Check sheet for the modelled part. Datum: model origin and axes. Units: mm. Coordinates: 2 decimals unless noted, no trailing zeros. Loops run counter-clockwise (first coordinate to the right, second up) from the corner with the lowest first, then second, coordinate; pieces in that order, holes last. Notation, with made-up numbers: (17, 29) - (60, 29) arc R23 ccw to (60, 49) - close; hole circle Ø6 at (17.5, -22). An arc over 180 degrees is marked (long way). Write each question's results on one line, items separated by ' | '. Start each with the question number.
1. Cross-section at A-A (x = 11.5). Record the cut outline in (y, z), and give its area (3 significant figures).
2. Thickness scan on line 1 (Z direction, x = 4, y = 6.5); line 2 (Z direction, x = 10, y = 7); line 3 (X direction, y = 3.75, z = -44.5). Record the ranges inside material, lowest first. Write a range as [from, to].
3. Cross-section at C-C (y = 3.75). Record the cut outline in (x, z).
4. Cross-section at B-B (z = -42). Record the cut outline in (x, y).
5. Cross-section at D-D (x = 3.5). Record the cut outline in (y, z), and give its area (3 significant figures).
```python
from build123d import *

# Parameters (mm, degrees)
SKETCH1_R           = 7
BOSS_EXTRUDE1_DEPTH = 8


with BuildPart() as part:
    # Sketch1 → Boss-Extrude1 (new body)
    with BuildSketch(Plane(origin=(0, 0, 0), x_dir=(1, 0, 0), z_dir=(0, 1, 0))):
        with BuildLine():
            Line((45.232378219, 82.321586231), (45.232378219, -94.678413769))
            Line((45.232378219, -94.678413769), (-13.267621781, -94.678413769))
            ThreePointArc((-13.267621781, -94.678413769), (-18.924476031, -92.335268019), (-21.267621781, -86.678413769))
            Line((-21.267621781, -86.678413769), (-21.267621781, 74.321586231))
            ThreePointArc((-21.267621781, 74.321586231), (-18.924476031, 79.97844048), (-13.267621781, 82.321586231))
            Line((-13.267621781, 82.321586231), (45.232378219, 82.321586231))
        make_face()
        with Locations(Location((7.732378219, -56.178413769, 0), (0, 0, 270))):
            Circle(SKETCH1_R, mode=Mode.SUBTRACT)
        with Locations(Location((7.732378219, 43.821586231, 0), (0, 0, 270))):
            Circle(SKETCH1_R, mode=Mode.SUBTRACT)
    extrude(amount=BOSS_EXTRUDE1_DEPTH)


solid = part.part
```
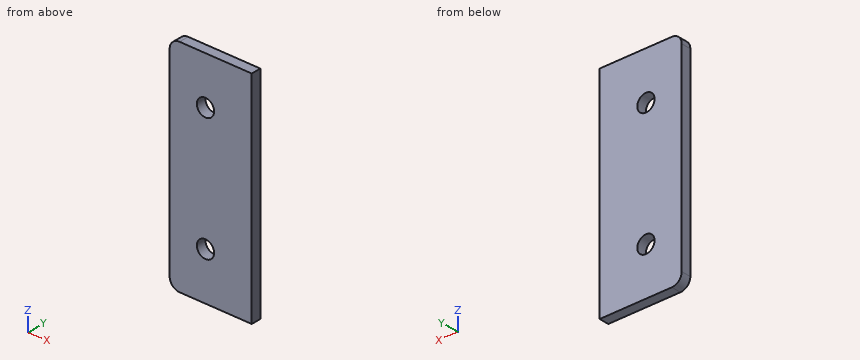
Established:
1) outline: (0, -82.32) - (8, -82.32) - (8, -49.72) - (0, -49.72) - close; (0, -37.92) - (8, -37.92) - (8, 50.28) - (0, 50.28) - close; (0, 62.08) - (8, 62.08) - (8, 94.68) - (0, 94.68) - close | area: 1,230 mm^2
2) line 1: [-82.32, -49.74], [-37.9, 50.26], [62.1, 94.68] | line 2: [-82.32, -50.44], [-37.2, 49.56], [62.8, 94.68] | line 3: [-21.27, 0.77], [14.7, 45.23]
3) outline: (-21.27, -74.32) arc R8 ccw to (-13.27, -82.32) - (45.23, -82.32) - (45.23, 94.68) - (-13.27, 94.68) arc R8 ccw to (-21.27, 86.68) - close; hole circle Ø14 at (7.73, -43.82); hole circle Ø14 at (7.73, 56.18)
4) outline: (-21.27, 0) - (0.97, 0) - (0.97, 8) - (-21.27, 8) - close; (14.49, 0) - (45.23, 0) - (45.23, 8) - (14.49, 8) - close
5) outline: (0, -82.32) - (8, -82.32) - (8, -49.4) - (0, -49.4) - close; (0, -38.25) - (8, -38.25) - (8, 50.6) - (0, 50.6) - close; (0, 61.75) - (8, 61.75) - (8, 94.68) - (0, 94.68) - close | area: 1,240 mm^2
